The drawing under review shows one solid part. Ordinate dimensions are in mm from its lowest x, y, z. Coordinates: 2 decimals unless noted, no trailing zeros. Order: outer loops, then holes, each group sorted by start corner. A loop starts at its lowest first (then second) coordinate and runs counter-clockwise, first axis right, second up.
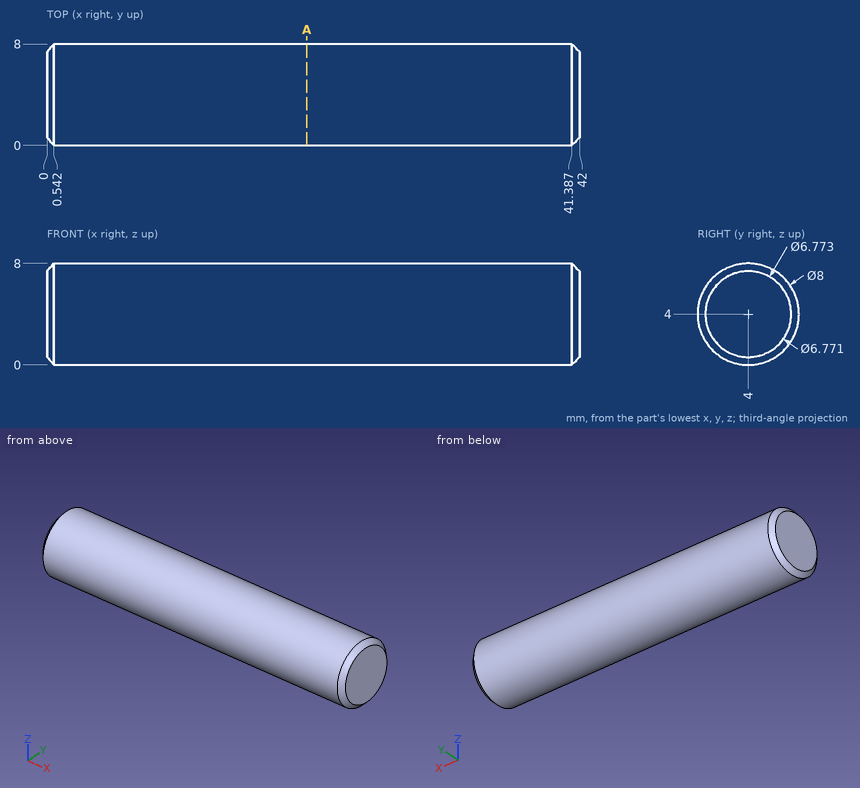
(1) Wall thickness on probe 1 along Y at (x, z) = (18, 1.5); probe 2 along Y at (x, z) = (20.5, 0.5) (1 decimal); probe 3 along Z at (x, y) = (35.5, 2) (1 decimal): over which ranges is each line inside the solid? List them lowest first.
A:
probe 1: y = 0.88 to 7.12
probe 2: y = 2.1 to 5.9
probe 3: z = 0.5 to 7.5
(2) For pin 1 Ø2 at (y, z) = (6.5, 7) entering from +X; pin 2 Ø1.5 at (x, z) = (21, 1.5) entering from +Y, all flat-tipped, find the tip position at first contact; note any pin that passes through.
A:
pin 1: stops at x = 42
pin 2: stops at y = 7.6
(3) We need section A-A, the plane x = 20.5. Write out the cut boundary in (y, z).
A:
outline: circle Ø8 at (4, 4)
